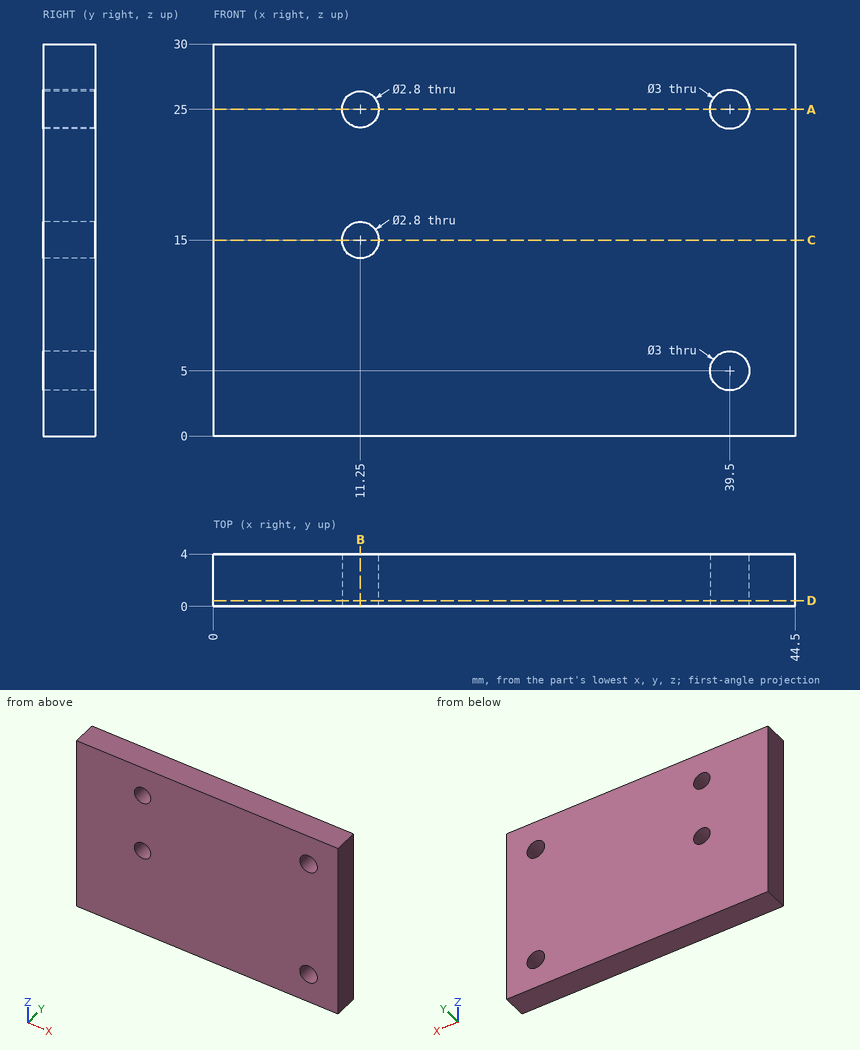
Study the drawing (mm; zero at the part's minimum x, y, z) and answer. Give positions to 0.01 mm unless a question says otherwise; leave off trailing zeros. Order: outer loops, then holes, each group sorted by start corner. A loop starts at its lowest first (then second) coordinate and runs counter-clockwise, first axis right, second up.
1) Given P1, Ø10, axis at x = 25.5, z = 22.5, coming from the -Y side; P2, Ø2, axis at x = 11.25, z = 25, coming from the +Y side, each flat-ended and moving along its own axis, determine where each tip first touches the part or whether it passes through.
Reported:
P1: stops at y = 0
P2: passes through
2) Find section C-C on z = 15. Write down the section's boundary in (x, y).
Reported:
outline: (0, 0) - (9.85, 0) - (9.85, 4) - (0, 4) - close; (12.65, 0) - (44.5, 0) - (44.5, 4) - (12.65, 4) - close
3) Find section A-A on z = 25. Write down the section's boundary in (x, y), then the cut area to 3 significant figures.
Reported:
outline: (0, 0) - (9.85, 0) - (9.85, 4) - (0, 4) - close; (12.65, 0) - (38, 0) - (38, 4) - (12.65, 4) - close; (41, 0) - (44.5, 0) - (44.5, 4) - (41, 4) - close
area: 155 mm2
4) Consider line 1 along Z through (x, y) = (39.5, 1.4); line 2 along Z through (x, y) = (11.25, 1.15); line 3 along X through (y, z) = (2.45, 25.5). Determine where each line is inside the solid, lowest interval first.
Reported:
line 1: z = 0 to 3.5, 6.5 to 23.5, 26.5 to 30
line 2: z = 0 to 13.6, 16.4 to 23.6, 26.4 to 30
line 3: x = 0 to 9.94, 12.56 to 38.09, 40.91 to 44.5
5) Find section D-D on y = 0.45. Write down the section's boundary in (x, z).
Reported:
outline: (0, 0) - (44.5, 0) - (44.5, 30) - (0, 30) - close; hole circle Ø2.8 at (11.25, 15); hole circle Ø2.8 at (11.25, 25); hole circle Ø3 at (39.5, 5); hole circle Ø3 at (39.5, 25)
6) Find section B-B on x = 11.25. Write down the section's boundary in (y, z).
Reported:
outline: (0, 0) - (4, 0) - (4, 13.6) - (0, 13.6) - close; (0, 16.4) - (4, 16.4) - (4, 23.6) - (0, 23.6) - close; (0, 26.4) - (4, 26.4) - (4, 30) - (0, 30) - close
